Here's the drawing with two shaded views (mm, measured from the low corner). I have some questions. Give positions to 0.01 mm unless a question says otherwise; leave off trailing zeros. Loops run counter-clockwise (first coordinate to the right, second up) from the corner with the lowest first, then second, coordinate; pieces in that order, holes last. Notation, with made-up numbers: (4.25, 48) -> (30.25, 48) arc R17 cw to (30.25, 69) -> close; hole circle Ø6 at (74.5, 85). An arc over 180 degrees is marked (long way). Answer in a Markdown table with one row per item. Add a question column.
Item 1: If we section it at A-A (y = 11.25): Write out the boundary of the cut face in (x, z).
Item 2: If I drill on line 1 (X direction, y = 10.25, z = 9); line 2 (X direction, y = 12.25, z = 5); line 3 (Z direction, x = 12, y = 10) (1 decimal), over which ranges is the centre line in solid material (lowest first)?
Item 3: For P1, Ø5, axis at x = 13.5, z = 7.5, coming from the +Y side; P2, Ø4, axis at y = 5.5, z = 3, coming from the +X side; P3, Ø1.6, axis at x = 8.5, z = 9, coming from the +Y side; P4, Ø1.5, axis at x = 4, y = 12.5, coming from the +Z side, each with a flat end and sliding along its axis, tell me the tip position at first contact or that it passes through.
Item 4: If we section it at B-B (y = 1.25): Write out the boundary of the cut face in (x, z), then the cut area to 3 significant figures.
Item 5: We'd pull the mould along Z, two halves only. Please class the marked faces 1, 2 and 3: released by +Z, released by -Z, zero draft, split by the parting line, or undercut.
Item 6: If we section it at C-C (y = 3): Write out the boundary of the cut face in (x, z).
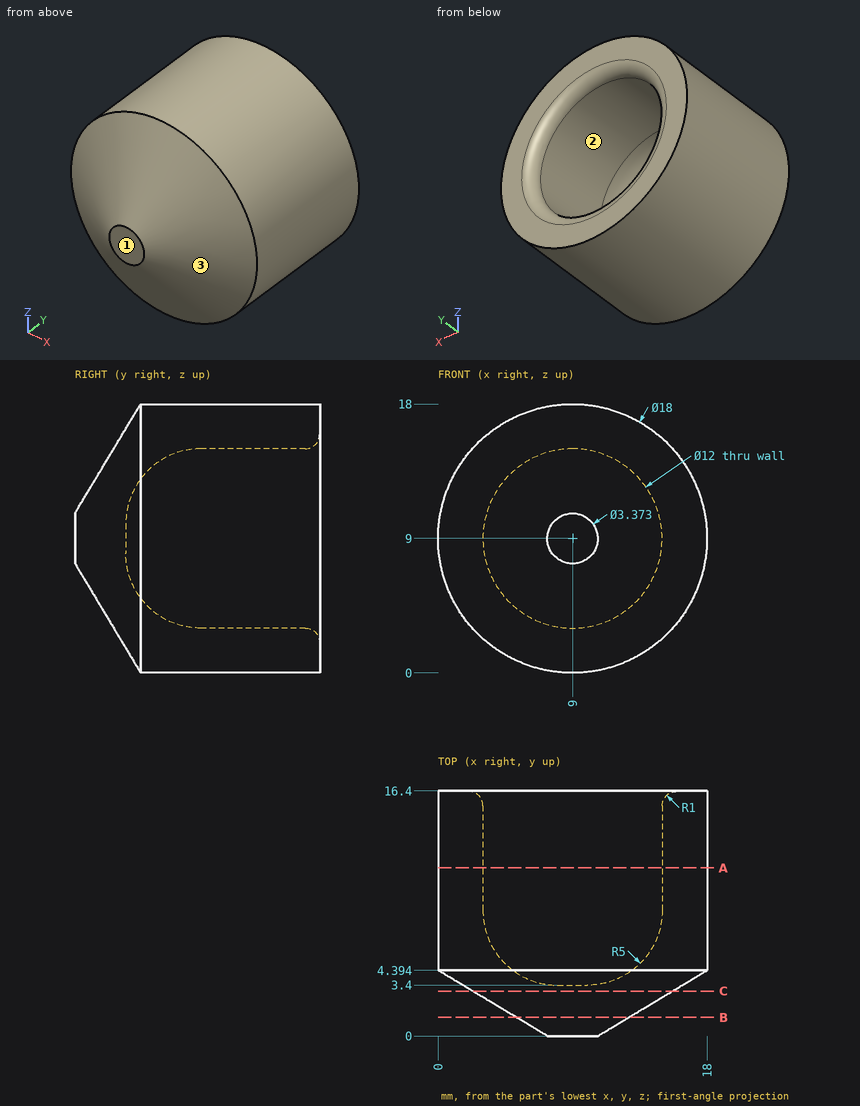
Recorded:
| question | item | result |
|---|---|---|
| 1 | outline | circle Ø18 at (9, 9); hole circle Ø12 at (9, 9) |
| 2 | line 1 | x = 0 to 3, 15 to 18 |
| 2 | line 2 | x = 0.94 to 4.53, 13.47 to 17.06 |
| 2 | line 3 | z = 0.5 to 3.8, 14.2 to 17.5 |
| 3 | P1 | stops at y = 16.4 |
| 3 | P2 | stops at x = 17.06 |
| 3 | P3 | stops at y = 3.41 |
| 3 | P4 | stops at z = 16.93 |
| 4 | outline | circle Ø7.53 at (9, 9) |
| 4 | area | 44.6 mm^2 |
| 5 | face 1 | zero draft |
| 5 | face 2 | undercut |
| 5 | face 3 | split by the parting line |
| 6 | outline | circle Ø13.36 at (9, 9) |
